Work out the finished part from the listing and answer in its coordinate system (mm). Face numbers are marked on the shaded views. A direction names the side the tool comes from. Give positions to 0.01 mm unless a question says otherwise; leave off trailing zeros. Loops run counter-clockwise (first coordinate to the right, second up) from the corner with the lowest first, then second, coordinate; pieces in that order, holes last. Notation, with made-up numbers: M 62.25,55.25 L 74.25,55.25 A17 cw 74.25,67.25 Z; hole C -37.5,-36.5 d8. An arc over 180 degrees is marked long. Use a Markdown table: item, result.
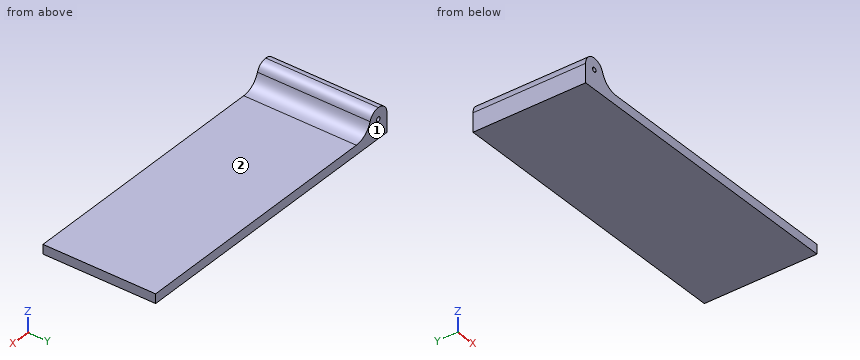
```python
from build123d import *

# Parameters (mm, degrees)
BOSS_EXTRUDE1_DEPTH = 30
FILLET1_R           = 5


with BuildPart() as part:
    # Sketch1 → Boss-Extrude1 (new body)
    with BuildSketch(Plane(origin=(0, 0, 0), x_dir=(1, 0, 0), z_dir=(0, 1, 0))):
        with BuildLine():
            Line((80, 0), (3, 0))
            Line((3, 0), (3, -2))
            ThreePointArc((3, -2), (3.866025404, -2.127718677), (4.658312395, -2.5))
            Line((4.658312395, -2.5), (80, -2.5))
            Line((80, -2.5), (80, 0))
        make_face()
        with BuildLine():
            Line((3, -2), (3, 0))
            Line((3, 0), (0, 0))
            Line((0, 0), (0, -2.5))
            Line((0, -2.5), (1.341687605, -2.5))
            ThreePointArc((1.341687605, -2.5), (2.133974596, -2.127718677), (3, -2))
        make_face()
        with BuildLine():
            ThreePointArc((0, -5), (0.356617963, -3.581362835), (1.341687605, -2.5))
            Line((1.341687605, -2.5), (0, -2.5))
            Line((0, -2.5), (0, -5))
        make_face()
        with BuildLine():
            Line((3, -4.4), (3, -2.5))
            Line((3, -2.5), (0, -5))
            ThreePointArc((0, -5), (0.878679656, -7.121320344), (3, -8))
            Line((3, -8), (3, -5.6))
            ThreePointArc((3, -5.6), (2.4, -5), (3, -4.4))
        make_face()
        with BuildLine():
            Line((4.658312395, -2.5), (3, -2.5))
            Line((3, -2.5), (3, -4.4))
            ThreePointArc((3, -4.4), (3.424264069, -4.575735931), (3.6, -5))
            ThreePointArc((3.6, -5), (3.424264069, -5.424264069), (3, -5.6))
            Line((3, -5.6), (3, -8))
            ThreePointArc((3, -8), (5.121320344, -7.121320344), (6, -5))
            ThreePointArc((6, -5), (5.643382037, -3.581362835), (4.658312395, -2.5))
        make_face()
        with BuildLine():
            Line((0, -5), (3, -2.5))
            Line((3, -2.5), (1.341687605, -2.5))
            ThreePointArc((1.341687605, -2.5), (0.356617963, -3.581362835), (0, -5))
        make_face()
        with BuildLine():
            Line((3, -2.5), (3, -2))
            ThreePointArc((3, -2), (2.133974596, -2.127718677), (1.341687605, -2.5))
            Line((1.341687605, -2.5), (3, -2.5))
        make_face()
        with BuildLine():
            ThreePointArc((4.658312395, -2.5), (3.866025404, -2.127718677), (3, -2))
            Line((3, -2), (3, -2.5))
            Line((3, -2.5), (4.658312395, -2.5))
        make_face()
    extrude(amount=BOSS_EXTRUDE1_DEPTH)

    # Fillet1
    fillet1_edges = [part.edges().sort_by_distance(p)[0] for p in [
        (4.658312395, 15, 2.5),
    ]]
    fillet(fillet1_edges, radius=FILLET1_R)


solid = part.part
```
(1) Which of the six approach directions +Z, -Z, +X, -X, +Y, -Y give full straight-line access (tool end or side, diameter ignored) to the marked faces 1 and 2?
Entries:
| item | result |
|---|---|
| face 1 | +Z, -Z, +X, -X, +Y |
| face 2 | +Z, +X, +Y, -Y |
(2) A cutting plane is placed at A-A (x = 34.5). Write down the section's boundary in (y, z).
Entries:
| item | result |
|---|---|
| outline | M 0,0 L 30,0 L 30,2.5 L 0,2.5 Z |
(3) Given P1, Ø2, axis at y = 6, z = 6, coming from the +X side; P2, Ø3, axis at y = 19, z = 5, coming from the +X side; P3, Ø9, axis at x = 49.5, y = 8, coming from the +Z side, each flat-ended and moving along its own axis, determine where each tip first touches the part or whether it passes through.
Entries:
| item | result |
|---|---|
| P1 | stops at x = 6.27 |
| P2 | stops at x = 7.6 |
| P3 | stops at z = 2.5 |
(4) Consider probe 1 along Z at (x, y) = (37.5, 22.5); probe 2 along X at (y, z) = (7, 4.5); probe 3 along X at (y, z) = (10, 5). Determine where each line is inside the solid, lowest interval first. Write a range as [from, to].
Entries:
| item | result |
|---|---|
| probe 1 | z = [0, 2.5] |
| probe 2 | x = [0, 2.67], [3.33, 6.6] |
| probe 3 | x = [0, 2.4], [3.6, 6.27] |
